from build123d import *

# Parameters (mm, degrees)
SKETCH1_R           = 6.35
BOSS_EXTRUDE1_DEPTH = 5.08
SKETCH2_R           = 2.545711461
CUT_EXTRUDE1_DEPTH  = 5.08
CUT_EXTRUDE4_DEPTH  = 5.08


with BuildPart() as part:
    # Sketch1 → Boss-Extrude1 (new body)
    with BuildSketch(Plane.XY):
        Circle(SKETCH1_R)
    extrude(amount=BOSS_EXTRUDE1_DEPTH)

    # Sketch2 → Cut-Extrude1 (cut)
    with BuildSketch(Plane.XY.offset(5.08)):
        Circle(SKETCH2_R)
    extrude(amount=-CUT_EXTRUDE1_DEPTH, mode=Mode.SUBTRACT)

    # Sketch6 → Cut-Extrude4 (cut)
    with BuildSketch(Plane(origin=(0, 0, 0), x_dir=(-1, 0, 0), z_dir=(0, 0, -1))):
        with BuildLine():
            Line((-6.313419859, 0.680609785), (-4.841727293, 1.082552663))
            ThreePointArc((-4.841727293, 1.082552663), (-4.737782551, 1.472297507), (-4.602520026, 1.852310143))
            Line((-4.602520026, 1.852310143), (-5.544711841, 3.094942746))
            ThreePointArc((-5.544711841, 3.094942746), (-6.050708452, 1.926506484), (-6.313419859, 0.680609785))
        make_face()
        with BuildLine():
            ThreePointArc((-4.621895526, -1.803420416), (-4.697643554, -1.595740734), (-4.764064977, -1.384892901))
            Line((-4.764064977, -1.384892901), (-6.284089397, -0.912535181))
            ThreePointArc((-6.284089397, -0.912535181), (-6.095179755, -1.780809857), (-5.786915427, -2.614213043))
            Line((-5.786915427, -2.614213043), (-4.621895526, -1.803420416))
        make_face()
        with BuildLine():
            ThreePointArc((-2.49633596, -4.287487636), (-2.747933203, -4.130751331), (-2.989720929, -3.959269152))
            Line((-2.989720929, -3.959269152), (-4.414172057, -4.564820375))
            ThreePointArc((-4.414172057, -4.564820375), (-3.704724213, -5.157278207), (-2.916783485, -5.640467543))
            Line((-2.916783485, -5.640467543), (-2.49633596, -4.287487636))
        make_face()
        with BuildLine():
            ThreePointArc((0.658971441, -4.91731635), (0.164985262, -4.958530358), (-0.330647946, -4.950243972))
            Line((-0.330647946, -4.950243972), (-0.797062617, -6.299777074))
            ThreePointArc((-0.797062617, -6.299777074), (0.162157154, -6.347929194), (1.117667403, -6.250865506))
            Line((1.117667403, -6.250865506), (0.658971441, -4.91731635))
        make_face()
        with BuildLine():
            ThreePointArc((3.079848524, -3.889572794), (2.834017843, -4.072172186), (2.577390132, -4.23925743))
            Line((2.577390132, -4.23925743), (2.695058949, -5.74970932))
            ThreePointArc((2.695058949, -5.74970932), (3.630700167, -5.209656063), (4.461255519, -4.518816127))
            Line((4.461255519, -4.518816127), (3.079848524, -3.889572794))
        make_face()
        with BuildLine():
            ThreePointArc((4.764064977, -1.384892901), (4.689120213, -1.620615648), (4.602520026, -1.852310143))
            Line((4.602520026, -1.852310143), (5.609586886, -2.975741079))
            ThreePointArc((5.609586886, -2.975741079), (6.026210342, -2.001821398), (6.2751364, -0.972195025))
            Line((6.2751364, -0.972195025), (4.764064977, -1.384892901))
        make_face()
        with BuildLine():
            ThreePointArc((4.697742855, 1.595448377), (4.785985372, 1.307129477), (4.856550498, 1.013982598))
            Line((4.856550498, 1.013982598), (6.301072583, 0.786755552))
            ThreePointArc((6.301072583, 0.786755552), (6.117140529, 1.703846165), (5.800483524, 2.583968051))
            Line((5.800483524, 2.583968051), (4.697742855, 1.595448377))
        make_face()
        with BuildLine():
            Line((-4.631054346, 4.34463297), (-3.274854363, 3.726871658))
            ThreePointArc((-3.274854363, 3.726871658), (-2.997527533, 3.953362131), (-2.704587495, 4.159260744))
            Line((-2.704587495, 4.159260744), (-2.823654461, 5.68765993))
            ThreePointArc((-2.823654461, 5.68765993), (-3.787360718, 5.096900901), (-4.631054346, 4.34463297))
        make_face()
        with BuildLine():
            Line((-1.15729269, 6.243650665), (-0.330647946, 4.950243972))
            ThreePointArc((-0.330647946, 4.950243972), (0.099169547, 4.960283142), (0.528242314, 4.933072421))
            Line((0.528242314, 4.933072421), (1.127688946, 6.249065341))
            ThreePointArc((1.127688946, 6.249065341), (-0.015047428, 6.349982171), (-1.15729269, 6.243650665))
        make_face()
        with BuildLine():
            Line((2.80655769, 5.696115688), (2.577390132, 4.23925743))
            ThreePointArc((2.577390132, 4.23925743), (2.937316156, 3.998301796), (3.274854363, 3.726871658))
            Line((3.274854363, 3.726871658), (4.557114361, 4.422127169))
            ThreePointArc((4.557114361, 4.422127169), (3.736532912, 5.134279092), (2.80655769, 5.696115688))
        make_face()
    extrude(amount=-CUT_EXTRUDE4_DEPTH, mode=Mode.SUBTRACT)


solid = part.part
Check sheet for the modelled part. Datum: model origin and axes. Units: mm. A direction names the side the tool comes from. Give positions to 0.01 mm unless a question says otherwise; leave off trailing zeros. Order: outer loops, then holes, each group sorted by start corner. A loop starts at its lowest first (then second) coordinate and runs counter-clockwise, first axis right, second up. Notation, with made-up numbers: M 37.5,23.5 L 69.5,23.5 A15 cw 69.5,34.5 Z; hole C -10,73.25 d9. An arc over 180 degrees is marked long. Answer as CSV lines item,"result". Start each with the question number.
Item 1: Mould release check, pull along X, two halves, no side actions. Record for faces 1 (the face through (-5.1, -3.78, 2.5)), 2 (the face through (5.067, 2.465, 2.504)), 3 (the face through (-0.824, 5.582, 2.504)), 4 (the face through (1, 6, 3)): +X half, -X half, draft (parallel to the pull), parting line (faces both ways), or undercut.
Item 2: Cross-section at A-A on x = 0. Enter the section's corners in (y, z), plus the area to 3 significant figures.
Item 3: Cross-section at B-B on y = 0. Enter the section's corners in (x, z), plus the area to 3 significant figures.
Item 4: Gauge pin test, flat ends, axial feed: P1, Ø1, axis at y = -3.5, z = 1.5, coming from the +X side; P2, Ø1, axis at x = 2, z = 4, coming from the -Y side. Record the tip position at first contact, or that the pin passes through.
Item 5: Thickness scan on line 1 (Y direction, x = 5.25, z = 1); line 2 (X direction, y = -4, z = 3.05) (3 decimals); line 3 (Y direction, x = 0, z = 1.35). Record the ranges inside material, lowest first. Write a range as [from, to].
Item 6: Tool access check on faces 5 (the face through (2.71, -4.97, 2.5)), 6 (the face through (-5.57, 0.9, 2.5)), 7 (the face through (6, -1, 3)). Record the directions out of +Z, -Z, +X, -X, +Y, -Y that give a thin tool (end or side, any length) a straight path to the whole face; none if there is none.
Established:
1,face 1,"-X half"
1,face 2,"+X half"
1,face 3,"undercut"
1,face 4,"undercut"
2,outline,"M -4.96,0 L -2.55,0 L -2.55,5.08 L -4.96,5.08 Z; M 2.55,0 L 4.96,0 L 4.96,5.08 L 2.55,5.08 Z"
2,area,"24.5 mm^2"
3,outline,"M -6.35,0 L -2.55,0 L -2.55,5.08 L -6.35,5.08 Z; M 2.55,0 L 6.35,0 L 6.35,5.08 L 2.55,5.08 Z"
3,area,"38.7 mm^2"
4,P1,"stops at x = 5.6"
4,P2,"stops at y = -6.17"
5,line 1,"y = [-3.57, -2.24], [-1.23, 0.97], [2.71, 3.57]"
5,line 2,"x = [-4.932, -3.322], [-2.935, 2.935], [3.086, 4.932]"
5,line 3,"y = [-4.96, -2.55], [2.55, 4.96]"
6,face 5,"+Z, -Z"
6,face 6,"+Z, -Z, -X"
6,face 7,"+Z, -Z, +X"
